```python
from build123d import *

# Parameters (mm, degrees)
F0_W     = 110.979826
F0_H     = 93.036972
F1_DEPTH = 25.4
F2_R     = 17.443643
F3_DEPTH = 50.8
F6_DEPTH = 58.928


with BuildPart() as f1:
    # F0 (on Top) → F1 (new body)
    with BuildSketch(Plane.XY):
        Rectangle(F0_W, F0_H)
    extrude(amount=F1_DEPTH)

    # F2 (on face) → F3 (join)
    with BuildSketch(Plane.XY.offset(25.4)):
        Circle(F2_R)
    extrude(amount=F3_DEPTH)

    # F5 (on offset) → F6 (cut)
    with BuildSketch(Plane.XZ.offset(25.4)):
        Polygon((-31.497903, 79.689242), (-29.677777, 64.824864), (34.026667, 46.016887), (34.026667, 79.689242), align=None)
    extrude(amount=-F6_DEPTH, mode=Mode.SUBTRACT)


solid = f1.part
```
Read the model definition and answer for the solid it produces. Units are mm, in the model's axes. A direction names the side the tool comes from. Coordinates: 2 decimals unless noted, no trailing zeros. Write each loop counter-clockwise with the first axis right and the second up, starting at its lowest first coordinate (ties: lowest second). Pieces come first, ordered by that corner, then holes. Notation, with made-up numbers: (2, 46.25) - (28, 46.25) arc R24 cw to (28, 60.25) - close; hole circle Ø2 at (26.25, 13). An arc over 180 degrees is marked (long way). Answer as a JSON object with one key per item and string values. Group by question number.
1. A cutting plane is placed at C-C (z = 48). Determine the outline of the cut face in (x, y), plus the area to 3 significant figures.
2. A cutting plane is placed at A-A (y = 0). Determine the outline of the cut face in (x, z), plus the area to 3 significant figures.
3. Consider L1, parallel to Z at x = 30, y = 2; L2, parallel to X at y = -9, z = 40; L3, parallel to Z at x = -2, y = -8. Determine where each line is inside the solid, lowest interval first. Write a range as [from, to].
4. A cutting plane is placed at D-D (y = -36). Determine the outline of the cut face in (x, z).
5. Each of these flat-tipped pins is pushed along its axis until it touches: P1, Ø10, axis at x = -34.5, y = 14, coming from the +Z side; P2, Ø6, axis at x = 15.5, z = 31, coming from the +Y side; P3, Ø5, axis at y = 18, z = 41, coming from the -X side. Where does it stop, or does it pass through?
6. Which of the six approach directions +Z, -Z, +X, -X, +Y, -Y give full straight-line access (tool end or side, diameter ignored) to faces 1 (the flat face through (-1, 1, 0)), 2 (the flat face through (-1, 21, 25.4))?
7. A cutting plane is placed at B-B (x = 3). Determine the outline of the cut face in (y, z).
Worked out:
{
 "1": {"outline": "circle Ø34.89 at (0, 0)", "area": "956 mm²"},
 "2": {"outline": "(-55.49, 0) - (55.49, 0) - (55.49, 25.4) - (17.44, 25.4) - (17.44, 50.91) - (-17.44, 61.21) - (-17.44, 25.4) - (-55.49, 25.4) - close", "area": "3,890 mm²"},
 "3": {"L1": "z = [0, 25.4]", "L2": "x = [-14.94, 14.94]", "L3": "z = [0, 56.65]"},
 "4": {"outline": "(-55.49, 0) - (55.49, 0) - (55.49, 25.4) - (-55.49, 25.4) - close"},
 "5": {"P1": "stops at z = 25.4", "P2": "stops at y = 12.17", "P3": "stops at x = -8"},
 "6": {"face 1": "-Z, +X, -X, +Y, -Y", "face 2": "+Z"},
 "7": {"outline": "(-46.52, 0) - (46.52, 0) - (46.52, 25.4) - (17.18, 25.4) - (17.18, 55.18) - (-17.18, 55.18) - (-17.18, 25.4) - (-46.52, 25.4) - close"}
}
